Work out the finished part from the listing and answer in its coordinate system (mm). A direction names the side the tool comes from. Round coordinates to 2 decimals unless told otherwise and drop trailing zeros. Write each loop counter-clockwise with the first axis right and the second up, starting at its lowest first coordinate (ties: lowest second). Pieces come first, ordered by that corner, then holes. Notation, with made-up numbers: (81, 1.5) - (111, 1.5) arc R23 cw to (111, 35.5) - close; hole circle Ø7 at (57.25, 48.5). An arc over 180 degrees is marked (long way). Answer as a JSON object with one key per item and string values.
```python
from build123d import *

# Parameters (mm, degrees)
SKETCH1_W           = 22.84372425
SKETCH1_H           = 22.84372425
SKETCH1_R           = 1.7
BOSS_EXTRUDE1_DEPTH = 4
SKETCH2_W           = 22.84372425
SKETCH2_H           = 9.578137875
BOSS_EXTRUDE2_DEPTH = 4
SKETCH3_W           = 22.84372425
SKETCH3_H           = 4
BOSS_EXTRUDE3_DEPTH = 10
FILLET1_R           = 3


with BuildPart() as part:
    # Sketch1 → Boss-Extrude1 (new body)
    with BuildSketch(Plane.XY):
        Rectangle(SKETCH1_W, SKETCH1_H)
        with Locations((-8, 8)):
            Circle(SKETCH1_R, mode=Mode.SUBTRACT)
        with Locations((8, 8)):
            Circle(SKETCH1_R, mode=Mode.SUBTRACT)
        with Locations((8, -8)):
            Circle(SKETCH1_R, mode=Mode.SUBTRACT)
        with Locations((-8, -8)):
            Circle(SKETCH1_R, mode=Mode.SUBTRACT)
    extrude(amount=BOSS_EXTRUDE1_DEPTH)

    # Sketch2 → Boss-Extrude2 (add)
    with BuildSketch(Plane.XY):
        with Locations((0, -16.210931063)):
            Rectangle(SKETCH2_W, SKETCH2_H)
    extrude(amount=BOSS_EXTRUDE2_DEPTH)

    # Sketch3 → Boss-Extrude3 (add)
    with BuildSketch(Plane(origin=(0, 0, 0), x_dir=(-1, 0, 0), z_dir=(0, 0, -1))):
        with Locations((0, -19)):
            Rectangle(SKETCH3_W, SKETCH3_H)
    extrude(amount=BOSS_EXTRUDE3_DEPTH)

    # Fillet1
    fillet1_edges = [part.edges().sort_by_distance(p)[0] for p in [
        (0, -17, 0),
    ]]
    fillet(fillet1_edges, radius=FILLET1_R)


solid = part.part
```
Item 1: For faces 1 (the flat face through (0, -1, 0)), 2 (the flat face through (0, -21, -3)), determine the directions among +Z, -Z, +X, -X, +Y, -Y from which every point of the face is accessible in a straight line to the end or side of a thin tool.
Results found:
{"face 1": "-Z, +X, -X, +Y", "face 2": "+Z, -Z, +X, -X, -Y"}
Item 2: A cutting plane is placed at C-C (y = 8). Write down the section's boundary in (x, z), and give its area (3 significant figures).
Results found:
{"outline": "(-11.42, 0) - (-9.7, 0) - (-9.7, 4) - (-11.42, 4) - close; (-6.3, 0) - (6.3, 0) - (6.3, 4) - (-6.3, 4) - close; (9.7, 0) - (11.42, 0) - (11.42, 4) - (9.7, 4) - close", "area": "64.2 mm²"}
Item 3: A cutting plane is placed at B-B (z = 2). Write down the section's boundary in (x, y), and give its area (3 significant figures).
Results found:
{"outline": "(-11.42, -21) - (11.42, -21) - (11.42, 11.42) - (-11.42, 11.42) - close; hole circle Ø3.4 at (-8, -8); hole circle Ø3.4 at (-8, 8); hole circle Ø3.4 at (8, -8); hole circle Ø3.4 at (8, 8)", "area": "704 mm²"}
Item 4: Each of these flat-tipped pins is pushed along its axis until it touches: P1, Ø5.5, axis at x = -8, y = -8, coming from the -Z side; P2, Ø2.5, axis at x = -8, y = 8, coming from the -Z side (3 decimals); P3, Ø5.5, axis at x = 2.5, z = -5, coming from the +Y side; P4, Ø1, axis at x = 2, z = -3.5, coming from the +Y side. Where does it stop, or does it pass through?
Results found:
{"P1": "z = 0", "P2": "through", "P3": "y = -16.9", "P4": "y = -17"}
Item 5: A cutting plane is placed at D-D (x = 0.75). Write down the section's boundary in (y, z).
Results found:
{"outline": "(-21, -10) - (-17, -10) - (-17, -3) arc R3 cw to (-14, 0) - (11.42, 0) - (11.42, 4) - (-21, 4) - close"}
Item 6: A cutting plane is placed at A-A (x = 8). Write down the section's boundary in (y, z), and give its area (3 significant figures).
Results found:
{"outline": "(-21, -10) - (-17, -10) - (-17, -3) arc R3 cw to (-14, 0) - (-9.7, 0) - (-9.7, 4) - (-21, 4) - close; (-6.3, 0) - (6.3, 0) - (6.3, 4) - (-6.3, 4) - close; (9.7, 0) - (11.42, 0) - (11.42, 4) - (9.7, 4) - close", "area": "144 mm²"}
Item 7: Consider line 1 along Y through (x, z) = (-8, 1.2); line 2 along Y through (x, z) = (7, 2.75); line 3 along Z through (x, y) = (1, -10). Determine where each line is inside the solid, lowest interval first.
Results found:
{"line 1": "-21 to -9.7, -6.3 to 6.3, 9.7 to 11.42", "line 2": "-21 to -9.37, -6.63 to 6.63, 9.37 to 11.42", "line 3": "0 to 4"}
Item 8: Determine the mould class of faces 3 (the flat face through (-11.422, -8.6, 0.2)), 4 (the cylindrical face through (6.3, 8.07, 1.97)), 5 (the cylindrical face through (-0.16, -16.14, -0.9)) for opening direction Y: pulls with the +Y half, pulls with the -Y half, needs draft (parallel to the pull), parting line crosses it, or undercut.
Results found:
{"face 3": "needs draft", "face 4": "undercut", "face 5": "pulls with the +Y half"}
